Geometry: final body of the model. Coordinates: model frame, mm. Face numbers are marked on the shaded views. Round coordinates to 2 decimals unless told otherwise and drop trailing zeros. Loops run counter-clockwise (first coordinate to the right, second up) from the corner with the lowest first, then second, coordinate; pieces in that order, holes last. Notation, with made-up numbers: (41.5, 72.5) -> (99.5, 72.5) arc R24 ccw to (99.5, 89.5) -> close; hole circle Ø10 at (24, 33). An arc over 180 degrees is marked (long way). Answer in a Markdown table with one row per item.
```python
from build123d import *

# Parameters (mm, degrees)
ESBO_O1_R                  = 6
RESSALTO_EXTRUS_O1_DEPTH   = 3
FURO_DE_DI_METRO_3_0_3_1_D = 3
FURO_DE_DI_METRO_7_0_7_1_D = 7
FILETE1_R                  = 6


with BuildPart() as part:
    # Esboço1 → Ressalto-extrusão1 (new body)
    # profile 1 of 2: a face of its own
    with BuildSketch(Plane(origin=(0, 0, 0), x_dir=(1, 0, 0), z_dir=(0, 1, 0))):
        with Locations((13.8, 0)):
            Circle(ESBO_O1_R)
    # profile 2 of 2: a face of its own
    with BuildSketch(Plane(origin=(0, 0, 0), x_dir=(1, 0, 0), z_dir=(0, 1, 0))):
        with BuildLine():
            Line((0, 4), (48.9, 4))
            ThreePointArc((48.9, 4), (52.9, 0), (48.9, -4))
            Line((48.9, -4), (0, -4))
            ThreePointArc((0, -4), (-4, 0), (0, 4))
        make_face()
        with BuildLine():
            Line((0, 1), (3.7, 1))
            ThreePointArc((3.7, 1), (4.7, 0), (3.7, -1))
            Line((3.7, -1), (0, -1))
            ThreePointArc((0, -1), (-1, 0), (0, 1))
        make_face(mode=Mode.SUBTRACT)
        with BuildLine():
            Line((24.45, 1), (29.45, 1))
            ThreePointArc((29.45, 1), (30.45, 0), (29.45, -1))
            Line((29.45, -1), (24.45, -1))
            ThreePointArc((24.45, -1), (23.45, 0), (24.45, 1))
        make_face(mode=Mode.SUBTRACT)
    extrude(amount=RESSALTO_EXTRUS_O1_DEPTH)

    # Furo de diâmetro Ø3.0 (3)1 (through all)
    with Locations(Plane(origin=(0, 3, 0), x_dir=(1, 0, 0), z_dir=(0, 1, 0))):
        with Locations((48.9, 0)):
            Hole(FURO_DE_DI_METRO_3_0_3_1_D / 2)

    # Furo de diâmetro Ø7.0 (7)1 (through all)
    with Locations(Plane(origin=(0, 3, 0), x_dir=(1, 0, 0), z_dir=(0, 1, 0))):
        with Locations((13.8, 0)):
            Hole(FURO_DE_DI_METRO_7_0_7_1_D / 2)

    # Filete1
    filete1_edges = [part.edges().sort_by_distance(p)[0] for p in [
        (9.327864045, 1.5, -4),
        (18.272135955, 1.5, -4),
        (18.272135955, 1.5, 4),
        (9.327864045, 1.5, 4),
    ]]
    fillet(filete1_edges, radius=FILETE1_R)


solid = part.part
```
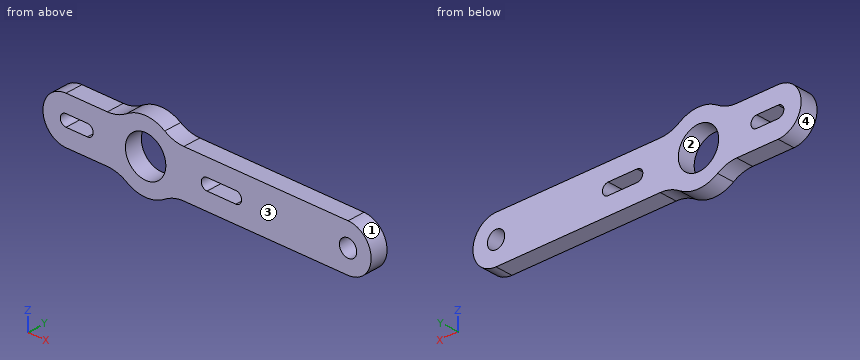
Item 1: First-contact query: P1, Ø1, axis at y = 1.5, z = 3.5, coming from the -X side; P2, Ø1, axis at x = 25.5, y = 1.5, coming from the -Z side; P3, Ø1.5, axis at x = 27.5, y = 1.5, coming from the +Z side. Flat tips, straight axial feed; report the tip coordinate or a pass-through.
Ans:
| item | result |
|---|---|
| P1 | x = -2.65 |
| P2 | z = -4 |
| P3 | z = 4 |
Item 2: Section query C-C, the plane y = 0.7. Output: boundary loops of the cut face in (x, z), and give its area (3 significant figures).
Ans:
| item | result |
|---|---|
| outline | (0, -4) -> (7.17, -4) arc R6 cw to (10.48, -5) arc R6 ccw to (17.12, -5) arc R6 cw to (20.43, -4) -> (48.9, -4) arc R4 ccw to (48.9, 4) -> (20.43, 4) arc R6 cw to (17.12, 5) arc R6 ccw to (10.48, 5) arc R6 cw to (7.17, 4) -> (0, 4) arc R4 ccw to start; hole (0, -1) -> (3.7, -1) arc R1 ccw to (3.7, 1) -> (0, 1) arc R1 ccw to start; hole circle Ø7 at (13.8, 0); hole (24.45, -1) -> (29.45, -1) arc R1 ccw to (29.45, 1) -> (24.45, 1) arc R1 ccw to start; hole circle Ø3 at (48.9, 0) |
| area | 399 mm2 |
Item 3: Section query D-D, the plane x = 13.8. Output: boundary loops of the cut face in (y, z).
Ans:
| item | result |
|---|---|
| outline | (0, -6) -> (3, -6) -> (3, -3.5) -> (0, -3.5) -> close; (0, 3.5) -> (3, 3.5) -> (3, 6) -> (0, 6) -> close |
Item 4: Mould query, pull axis X, two halves, no side actions, for the marked faces 1, 2, 3 and 4. Classes: released by +X, released by -X, zero draft, split by the parting line, or undercut.
Ans:
| item | result |
|---|---|
| face 1 | released by +X |
| face 2 | undercut |
| face 3 | zero draft |
| face 4 | released by -X |
Item 5: Ray query, L1, parallel to Z at x = 48.9, y = 0.7; L2, parallel to Z at x = 26, y = 0.5; L3, parallel to X at y = 1.3, z = -0.5. Return the intervals inside material, ascending.
Ans:
| item | result |
|---|---|
| L1 | -4 to -1.5, 1.5 to 4 |
| L2 | -4 to -1, 1 to 4 |
| L3 | -3.97 to -0.87, 4.57 to 10.34, 17.26 to 23.58, 30.32 to 47.49, 50.31 to 52.87 |
Item 6: Section query B-B, the plane z = 0. Output: boundary loops of the cut face in (x, y).
Ans:
| item | result |
|---|---|
| outline | (-4, 0) -> (-1, 0) -> (-1, 3) -> (-4, 3) -> close; (4.7, 0) -> (10.3, 0) -> (10.3, 3) -> (4.7, 3) -> close; (17.3, 0) -> (23.45, 0) -> (23.45, 3) -> (17.3, 3) -> close; (30.45, 0) -> (47.4, 0) -> (47.4, 3) -> (30.45, 3) -> close; (50.4, 0) -> (52.9, 0) -> (52.9, 3) -> (50.4, 3) -> close |
Item 7: Section query A-A, the plane x = 27. Output: boundary loops of the cut face in (y, z), and give its area (3 significant figures).
Ans:
| item | result |
|---|---|
| outline | (0, -4) -> (3, -4) -> (3, -1) -> (0, -1) -> close; (0, 1) -> (3, 1) -> (3, 4) -> (0, 4) -> close |
| area | 18.0 mm2 |
